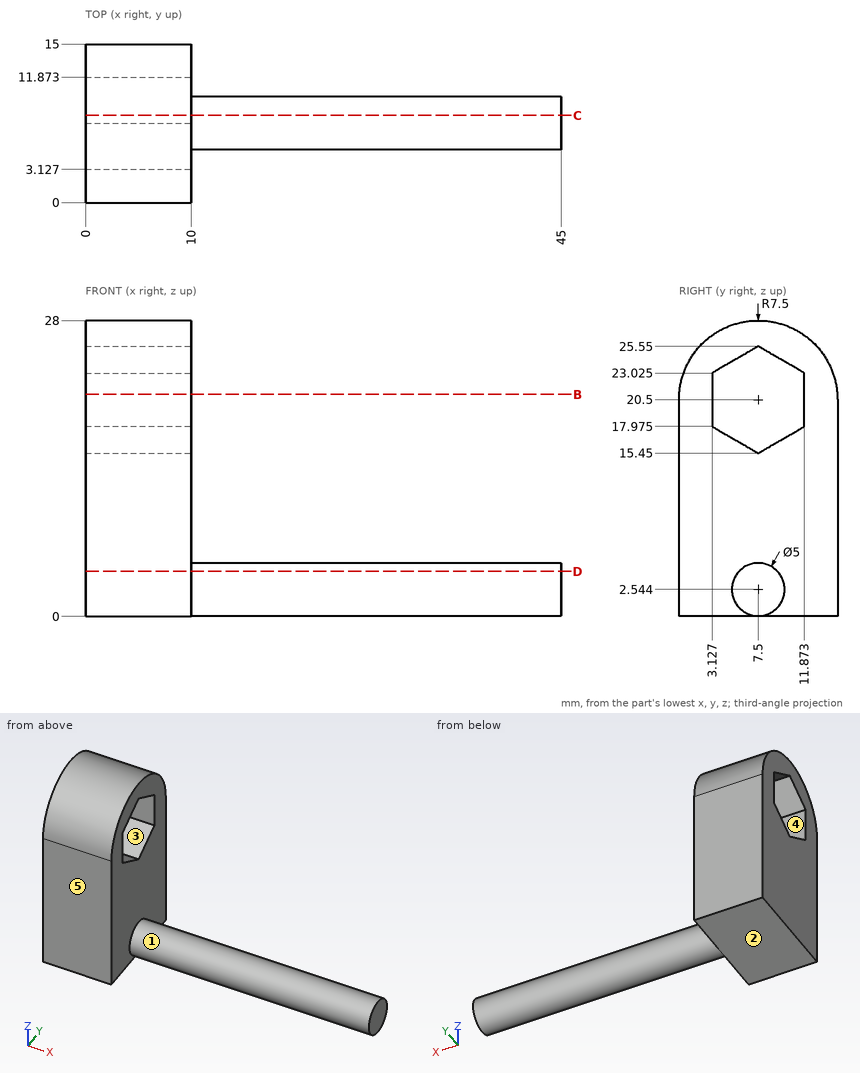
Can you work these out from the drawing? Everything is in mm from the part's minimum corner. A direction names the side the tool comes from. Round coordinates to 2 decimals unless told otherwise and drop trailing zeros. Order: outer loops, then holes, each group sorted by start corner. A loop starts at its lowest first (then second) coordinate and runs counter-clockwise, first axis right, second up. Notation, with made-up numbers: (-18, 7) -> (2, 7) arc R25 ccw to (2, 39) -> close; hole circle Ø2 at (-16, 47). An arc over 180 degrees is marked (long way). Use CSV: the item, a comma, the result in double quotes.
1. I want a section at D-D on z = 4.25. List the corners of the cut face in (x, y) for me.
Recorded:
outline,"(0, 0) -> (10, 0) -> (10, 5.67) -> (45, 5.67) -> (45, 9.33) -> (10, 9.33) -> (10, 15) -> (0, 15) -> close"
2. I want a section at B-B on z = 21. List the corners of the cut face in (x, y) for me, and give its area (3 significant figures).
Recorded:
outline,"(0, 0.02) -> (10, 0.02) -> (10, 3.13) -> (0, 3.13) -> close; (0, 11.87) -> (10, 11.87) -> (10, 14.98) -> (0, 14.98) -> close"
area,"62.2 mm2"
3. Which directions (+Z, -Z, +X, -X, +Y, -Y) give clear straight access to the entire face, cutting with the end or side of a thin tool? Please do the marked faces 4 and 5.
Recorded:
face 4,"+X, -X"
face 5,"+Z, -Z, +X, -X, -Y"
4. Thinking about a two-plate mould opening in Y: for the marked faces 1, 2 and 3, which applies, pulls with the +Y half, pulls with the -Y half, needs draft (parallel to the pull), parting line crosses it, or undercut?
Recorded:
face 1,"parting line crosses it"
face 2,"needs draft"
face 3,"undercut"
5. I'm going to push flat-ended pins straight in: P1, Ø4, axis at y = 9, z = 11, coming from the +X side; P2, Ø6, axis at x = 40, y = 5, coming from the -Z side; P3, Ø1.5, axis at x = 23.5, y = 4.5, coming from the -Z side (1 decimal). Where does each tip first touch, or does it pass through?
Recorded:
P1,"stops at x = 10"
P2,"stops at z = 0.04"
P3,"stops at z = 1.5"
6. I want a section at C-C on y = 8.25. List the corners of the cut face in (x, z) for me.
Recorded:
outline,"(0, 0) -> (10, 0) -> (10, 0.16) -> (45, 0.16) -> (45, 4.93) -> (10, 4.93) -> (10, 15.88) -> (0, 15.88) -> close; (0, 25.12) -> (10, 25.12) -> (10, 27.96) -> (0, 27.96) -> close"
7. I need wall thicknesses on line 1 along X through (y, z) = (9, 26.75); line 2 along Y through (x, z) = (12, 2.5); line 3 along Z through (x, y) = (5, 6.5). Which ranges of each line are inside material? Lowest first, please.
Recorded:
line 1,"x = 0 to 10"
line 2,"y = 5 to 10"
line 3,"z = 0 to 16.03, 24.97 to 27.93"
